Here's how the part is built. I have some questions about the finished solid (model axes, mm). Face numbers are marked on the shaded views. A direction names the side the tool comes from. Give positions to 0.01 mm unless a question says otherwise; leave off trailing zeros. Loops run counter-clockwise (first coordinate to the right, second up) from the corner with the lowest first, then second, coordinate; pieces in that order, holes last.
Q1. I need wall thicknesses on probe 1 along Y at (x, z) = (-14, -1.45); probe 2 along Z at (x, y) = (-6.25, 0.75); probe 3 along Z at (x, y) = (-1.15, 5). Which ranges of each line are inside material? Lowest first, please.
Q2. Suppose I cut it at C-C (y = 5). List the corners of the cut face in (x, z) for me, and give its area (3 significant figures).
Q3. Thinking about a two-plate mould opening in Z: for the marked faces 3, 4 and 5, which applies, pulls with the +Z half, pulls with the -Z half, needs draft (parallel to the pull), parting line crosses it, or undercut?
Q4. I'm going to push flat-ended pins straight in: P1, Ø3, axis at y = 5, z = -40, coming from the +X side; P2, Ø5, axis at y = 5.5, z = -34, coming from the -X side. Where does each tip first touch, or does it pass through?
Q5. Suppose I cut it at A-A (z = -12). List the corners of the cut face in (x, y) for me, and give its area (3 significant figures).
Q6. Suppose I cut it at B-B (x = -4.5). List the corners of the cut face in (y, z) for me.
Q7. Suppose I cut it at D-D (x = -14.75). List the corners of the cut face in (y, z) for me.
Q8. For the marked faces 1 and 2, which set-ups out of +Z, -Z, +X, -X, +Y, -Y let a thin tool reach every point of the face, with its end or its side?
Autodesk Inventor part; units mm, degrees
ref_plane "YZ Plane" through (0, 0, 0) normal (1, 0, 0) x (0, 1, 0)
ref_plane "XZ Plane" through (0, 0, 0) normal (0, 1, 0) x (-1, 0, 0)
ref_plane "XY Plane" through (0, 0, 0) normal (0, 0, 1) x (1, 0, 0)
sketch "Sketch1" plane through (0, 0, 0) normal (0, 1, 0) x (-1, 0, 0)
  line L0 (0, 0) -> (3, 0)
  line L1 (3, 0) -> (3, -52)
  line L2 (3, -52) -> (0, -52)
  line L3 (0, -52) -> (0, 0)
  line L4 (3, -52) -> (19, -52)
  line L5 (19, -52) -> (19, -49)
  line L6 (19, -49) -> (3, -49)
  line L7 (3, -49) -> (3, -52)
  line L8 (3, 0) -> (19, 0)
  line L9 (19, 0) -> (19, -3)
  line L10 (19, -3) -> (3, -3)
  line L11 (3, -3) -> (3, 0)
  dimension "d0" = 3
  dimension "d1" = 3
  dimension "d2" = 3
  dimension "d3" = 46
  dimension "d4" = 16
extrude "Extrusion1" add sketch "Sketch1" along normal blind 10
fillet "Fillet1" radius 1 2 edges at (-3, 5, -49) (-3, 5, -3)
fillet "Fillet2" radius 4 2 edges at (0, 5, -52) (0, 5, 0)
sketch "Sketch2" plane through (-19, 0, -52) normal (0, 0, -1) x (-1, 0, 0)
  line L0 (-15, 10) -> (0, 10)
  line L1 (0, 0) -> (0, 10)
  point P0 (-19, 0)
  point P1 (-5, 5)
  dimension "d9" = 5
  dimension "d10" = 5
hole "Hole1" at (-14, 5, -52) direction (0, 0, 1) diameter 3.4 end through all
sketch "Sketch3" plane through (0, 0, -4) normal (1, 0, 0) x (0, 0, -1)
  line L0 (44, 10) -> (44, 0)
  point P0 (-4, 0)
  point P1 (8, 5)
  point P2 (36, 5)
  point P3 (44, 5)
  point P4 (45, 10)
  point P5 (-1, 10)
  dimension "d18" = 9
  dimension "d19" = 9
hole "Hole2" at (0, 5, -12) at (0, 5, -40) direction (-1, 0, 0) diameter 3.4 end through all
equation "\"d1\" = d0"
equation "\"d2\" = d0"
properties part number "Top_End Stopper" material "Aluminum 6061"
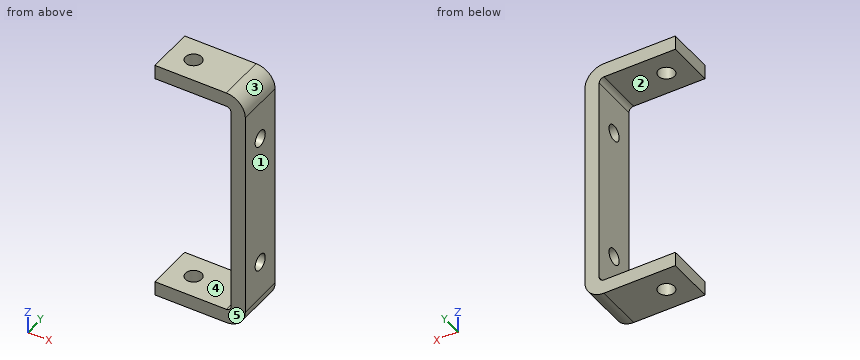
Solutions:
1. probe 1: y = 0 to 3.3, 6.7 to 10
1. probe 2: z = -52 to -49, -3 to 0
1. probe 3: z = -50.81 to -41.7, -38.3 to -13.7, -10.3 to -1.19
2. outline: (-19, -52) - (-15.7, -52) - (-15.7, -49) - (-19, -49) - close; (-19, -3) - (-15.7, -3) - (-15.7, 0) - (-19, 0) - close; (-12.3, -52) - (-4, -52) arc R4 ccw to (0, -48) - (0, -41.7) - (-3, -41.7) - (-3, -48) arc R1 cw to (-4, -49) - (-12.3, -49) - close; (-12.3, -3) - (-4, -3) arc R1 cw to (-3, -4) - (-3, -10.3) - (0, -10.3) - (0, -4) arc R4 ccw to (-4, 0) - (-12.3, 0) - close; (-3, -38.3) - (0, -38.3) - (0, -13.7) - (-3, -13.7) - close
2. area: 205 mm2
3. face 3: pulls with the +Z half
3. face 4: undercut
3. face 5: needs draft
4. P1: passes through
4. P2: stops at x = -3
5. outline: (-3, 0) - (0, 0) - (0, 3.3) - (-3, 3.3) - close; (-3, 6.7) - (0, 6.7) - (0, 10) - (-3, 10) - close
5. area: 19.8 mm2
6. outline: (0, -52) - (10, -52) - (10, -49) - (0, -49) - close; (0, -3) - (10, -3) - (10, 0) - (0, 0) - close
7. outline: (0, -52) - (3.47, -52) - (3.47, -49) - (0, -49) - close; (0, -3) - (3.47, -3) - (3.47, 0) - (0, 0) - close; (6.53, -52) - (10, -52) - (10, -49) - (6.53, -49) - close; (6.53, -3) - (10, -3) - (10, 0) - (6.53, 0) - close
8. face 1: +Z, -Z, +X, +Y, -Y
8. face 2: -X, +Y, -Y
